Here's how the part is built. I have some questions about the finished solid (model axes, mm). Face numbers are marked on the shaded views. A direction names the side the tool comes from. Coordinates: 2 decimals unless noted, no trailing zeros. Write each loop counter-clockwise with the first axis right and the second up, starting at its lowest first coordinate (ties: lowest second). Pieces come first, ordered by that corner, then holes. Notation, with made-up numbers: (20, -1.75) - (53, -1.75) arc R21 cw to (53, 3.25) - close; hole circle Ø5 at (-20, 19.25). An arc over 180 degrees is marked (long way). Answer in a Markdown table with one row per item. Add a question column.
Item 1: Imagine slicing it at A-A (y = -5.25). Please give me the cut outline in (x, z), plus the area to 3 significant figures.
Item 2: We'd pull the mould along X, two halves only. Please class the marked faces 1, 2, 3 and 4: +X half, -X half, draft (parallel to the pull), parting line (faces both ways), or undercut.
Item 3: Which directions (+Z, -Z, +X, -X, +Y, -Y) give clear straight access to the entire face, cutting with the end or side of a thin tool? Please do the marked faces 5, 6 and 7.
Item 4: I'm going to push flat-ended pins straight in: pin 1 (6 mm diameter, centred on x = -1, y = -6, fed in from -Z); pin 2 (4.5 mm diameter, centred on x = 1, z = -32.5, fed in from -Y); pin 3 (20.5 mm diameter, centred on x = -6.5, z = -26, fed in from +Y); pin 4 (9.5 mm diameter, centred on y = 2, z = -13.5, fed in from +X). Where does each tip first touch, or does it pass through?
Item 5: Imagine slicing it at B-B (z = 0). Please give me the cut outline in (x, y), plus the area to 3 significant figures.
Item 6: Imagine slicing it at C-C (x = 24). Please give me the cut outline in (y, z), plus the area to 3 significant figures.
Item 7: If I drill on probe 1 along Z at (x, y) = (0, -12.05); probe 2 along X at (y, z) = (-12.1, -25.4); probe 3 along Z at (x, y) = (-0.5, 1.5), over which ranges is the centre line in solid material (lowest first)? Write a range as from..to.
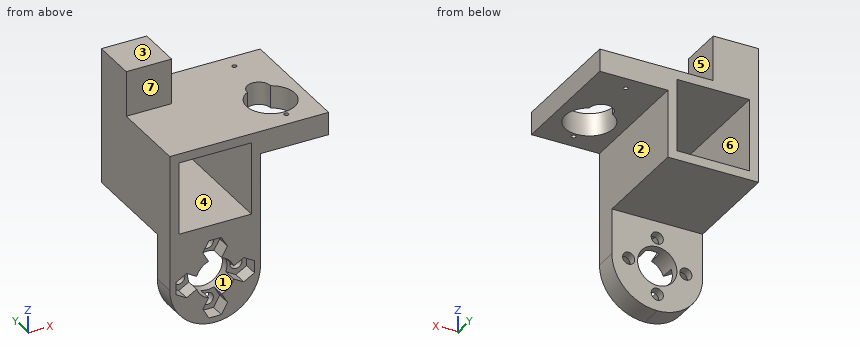
from build123d import *

# Parameters (mm, degrees)
SKETCH1_W            = 25.4
SKETCH1_H            = 25.4
SKETCH1_W_2          = 20.32
SKETCH1_H_2          = 20.32
BOSS_EXTRUDE1_DEPTH  = 17.4625
SKETCH4_W            = 25.4
SKETCH4_H            = 25.4
BOSS_EXTRUDE2_DEPTH  = 6.35
CUT_EXTRUDE1_REACH   = 51.289
SKETCH6_R            = 5.5
FILLET1_R            = 12.7
M3_CLEARANCE_HOLE1_D = 3.4
CIRPATTERN1_COUNT    = 4
CUT_EXTRUDE2_DEPTH   = 4
CIRPATTERN2_COUNT    = 4
SKETCH12_W           = 19.05
SKETCH12_H           = 34.925
BOSS_EXTRUDE3_DEPTH  = 6.35
SKETCH13_W           = 12.7
SKETCH13_H           = 12.7
BOSS_EXTRUDE4_DEPTH  = 12.7
CUT_EXTRUDE3_REACH   = 59.348
SKETCH15_R           = 0.635
CUT_EXTRUDE4_REACH   = 64.399


with BuildPart() as part:
    # Sketch1 → Boss-Extrude1 (new, symmetric)
    with BuildSketch(Plane(origin=(0, 0, 0), x_dir=(1, 0, 0), z_dir=(0, 1, 0))):
        Rectangle(SKETCH1_W, SKETCH1_H)
        Rectangle(SKETCH1_W_2, SKETCH1_H_2, mode=Mode.SUBTRACT)
    extrude(amount=BOSS_EXTRUDE1_DEPTH, both=True)

    # Sketch4 → Boss-Extrude2 (add)
    with BuildSketch(Plane.XZ.offset(17.4625)):
        with Locations((0, -25.4)):
            Rectangle(SKETCH4_W, SKETCH4_H)
    extrude(amount=-BOSS_EXTRUDE2_DEPTH)

    # Sketch6 → Cut-Extrude1 (cut, up to next)
    with BuildSketch(Plane(origin=(0, -11.1125, 0), x_dir=(1, 0, 0), z_dir=(0, 1, 0)), mode=Mode.PRIVATE) as cut_extrude1_sk1:
        with Locations(Location((0, 25.4, 0), (0, 0, 270))):
            Circle(SKETCH6_R)
    cut_extrude1_tool1 = extrude(cut_extrude1_sk1.sketch, amount=-CUT_EXTRUDE1_REACH, mode=Mode.PRIVATE) & part.part
    add(cut_extrude1_tool1.solids().sort_by_distance((0, -11.1125, -25.4))[0], mode=Mode.SUBTRACT)

    # Fillet1
    fillet1_edges = [part.edges().sort_by_distance(p)[0] for p in [
        (-12.7, -14.2875, -38.1),
        (12.7, -14.2875, -38.1),
    ]]
    fillet(fillet1_edges, radius=FILLET1_R - 0.0001)  # a hair under: the kernel refuses the full size

    # M3 Clearance Hole1 (through all)
    with Locations(Plane(origin=(0, -11.1125, 0), x_dir=(1, 0, 0), z_dir=(0, 1, 0))):
        with Locations((0, 33.4)):
            m3_clearance_hole1 = Hole(M3_CLEARANCE_HOLE1_D / 2)

    # CirPattern1: M3 Clearance Hole1 ×4 about axis
    cirpattern1_axis = Axis((0, 0, -25.4), (0, 1, 0))
    for i in range(1, CIRPATTERN1_COUNT):
        add(m3_clearance_hole1.rotate(cirpattern1_axis, i * 360 / CIRPATTERN1_COUNT), mode=Mode.SUBTRACT)

    # Sketch11 → Cut-Extrude2 (cut)
    with BuildSketch(Plane.XZ.offset(17.4625)):
        Polygon((1.732050808, -14.4), (-1.732050808, -14.4), (-3.464101615, -17.4), (-1.732050808, -20.4), (1.732050808, -20.4), (3.464101615, -17.4), align=None)
    cut_extrude2 = extrude(amount=-CUT_EXTRUDE2_DEPTH, mode=Mode.SUBTRACT)

    # CirPattern2: Cut-Extrude2 ×4 about axis
    cirpattern2_axis = Axis((0, 0, -25.4), (0, 1, 0))
    for i in range(1, CIRPATTERN2_COUNT):
        add(cut_extrude2.rotate(cirpattern2_axis, i * 360 / CIRPATTERN2_COUNT), mode=Mode.SUBTRACT)

    # Sketch12 → Boss-Extrude3 (add)
    with BuildSketch(Plane.XY.offset(12.7)):
        with Locations((22.225, 0)):
            Rectangle(SKETCH12_W, SKETCH12_H)
    extrude(amount=-BOSS_EXTRUDE3_DEPTH)

    # Sketch13 → Boss-Extrude4 (add)
    with BuildSketch(Plane.ZY.offset(12.7)):
        with Locations((19.05, 11.1125)):
            Rectangle(SKETCH13_W, SKETCH13_H)
    extrude(amount=-BOSS_EXTRUDE4_DEPTH)

    # Sketch15 → Cut-Extrude3 (cut, up to next)
    with BuildSketch(Plane(origin=(0, 0, 6.35), x_dir=(-1, 0, 0), z_dir=(0, 0, -1)), mode=Mode.PRIVATE) as cut_extrude3_sk1:
        with Locations((-22.225, 13.25)):
            Circle(SKETCH15_R)
    cut_extrude3_tool1 = extrude(cut_extrude3_sk1.sketch, amount=-CUT_EXTRUDE3_REACH, mode=Mode.PRIVATE) & part.part
    # Sketch15 → Cut-Extrude3 (cut, up to next)
    with BuildSketch(Plane(origin=(0, 0, 6.35), x_dir=(-1, 0, 0), z_dir=(0, 0, -1)), mode=Mode.PRIVATE) as cut_extrude3_sk2:
        with Locations((-22.225, -13.25)):
            Circle(SKETCH15_R)
    cut_extrude3_tool2 = extrude(cut_extrude3_sk2.sketch, amount=-CUT_EXTRUDE3_REACH, mode=Mode.PRIVATE) & part.part
    add(cut_extrude3_tool1.solids().sort_by_distance((22.225, 13.25, 6.35))[0], mode=Mode.SUBTRACT)
    add(cut_extrude3_tool2.solids().sort_by_distance((22.225, -13.25, 6.35))[0], mode=Mode.SUBTRACT)

    # Sketch16 → Cut-Extrude4 (cut, up to next)
    with BuildSketch(Plane.XY.offset(12.7), mode=Mode.PRIVATE) as cut_extrude4_sk1:
        with BuildLine():
            ThreePointArc((18.963893252, 0.673666667), (22.225, -12.012), (25.486106748, 0.673666667))
            ThreePointArc((25.486106748, 0.673666667), (22.225, 4.012), (18.963893252, 0.673666667))
        make_face()
    cut_extrude4_tool1 = extrude(cut_extrude4_sk1.sketch, amount=-CUT_EXTRUDE4_REACH, mode=Mode.PRIVATE) & part.part
    add(cut_extrude4_tool1.solids().sort_by_distance((22.225, -4.592909, 12.7))[0], mode=Mode.SUBTRACT)


solid = part.part
Here are the results:
| question | item | result |
|---|---|---|
| 1 | outline | (-12.7, -12.7) - (12.7, -12.7) - (12.7, 6.35) - (15.46, 6.35) - (15.46, 12.7) - (-12.7, 12.7) - close; (28.99, 6.35) - (31.75, 6.35) - (31.75, 12.7) - (28.99, 12.7) - close; hole (-10.16, -10.16) - (10.16, -10.16) - (10.16, 10.16) - (-10.16, 10.16) - close |
| 1 | area | 267 mm2 |
| 2 | face 1 | undercut |
| 2 | face 2 | +X half |
| 2 | face 3 | draft |
| 2 | face 4 | undercut |
| 3 | face 5 | +Z, +X, +Y, -Y |
| 3 | face 6 | +Y, -Y |
| 3 | face 7 | +Z, +X, -X, -Y |
| 4 | pin 1 | stops at z = -12.7 |
| 4 | pin 2 | stops at y = -17.46 |
| 4 | pin 3 | stops at y = -11.11 |
| 4 | pin 4 | stops at x = 12.7 |
| 5 | outline | (-12.7, -17.46) - (-10.16, -17.46) - (-10.16, 17.46) - (-12.7, 17.46) - close; (10.16, -17.46) - (12.7, -17.46) - (12.7, 17.46) - (10.16, 17.46) - close |
| 5 | area | 177 mm2 |
| 6 | outline | (-17.46, 6.35) - (-11.77, 6.35) - (-11.77, 12.7) - (-17.46, 12.7) - close; (3.49, 6.35) - (17.46, 6.35) - (17.46, 12.7) - (3.49, 12.7) - close |
| 6 | area | 125 mm2 |
| 7 | probe 1 | z = -38.1..-35.1, -31.7..-30.9, -19.9..-19.1, -15.7..-10.16, 10.16..12.7 |
| 7 | probe 2 | x = -12.7..-9.7, -6.3..-5.5, 5.5..6.3, 9.7..12.7 |
| 7 | probe 3 | z = -12.7..-10.16, 10.16..12.7 |
